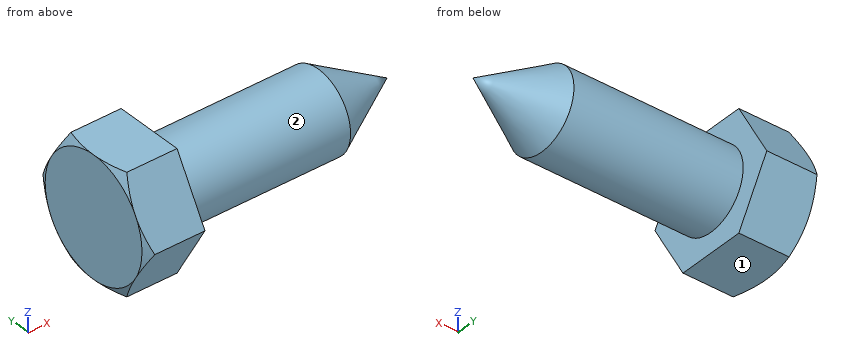
```python
from build123d import *

# Parameters (mm, degrees)
BASEHEAD_DEPTH = 17.78


with BuildPart() as part:
    # Sketch1 → BaseHead (new body)
    with BuildSketch(Plane(origin=(0, 0, 0), x_dir=(0, 0, -1), z_dir=(1, 0, 0))):
        Polygon((19.05, 10.998522628), (19.05, -10.998522628), (0, -21.997045256), (-19.05, -10.998522628), (-19.05, 10.998522628), (0, 21.997045256), align=None)
    extrude(amount=BASEHEAD_DEPTH)

    # Sketch2 → BaseBody (revolve)
    with BuildSketch(Plane.XY, mode=Mode.PRIVATE) as basebody_sk:
        Polygon((0, 0), (93.98, 0), (71.982954744, 12.7), (0, 12.7), align=None)
    revolve(basebody_sk.sketch.rotate(Axis((0, 0, 0), (1, 0, 0)), 90), axis=Axis((0, 0, 0), (1, 0, 0)))

    # Sketch3 → HeadChamfer (revolve, cut)
    with BuildSketch(Plane.XY):
        Polygon((0, 19.05), (5.367651581, 28.347045256), (5.367651581, 34.697045256), (-12.7, 34.697045256), (-12.7, 19.05), align=None)
    revolve(axis=Axis((0, 0, 0), (1, 0, 0)), mode=Mode.SUBTRACT)


solid = part.part
```
Input: part model. Units: mm. Frame: model coordinates. Face numbers are marked on the shaded views. A direction names the side the tool comes from. Coordinates: 2 decimals unless noted, no trailing zeros. Write each loop counter-clockwise with the first axis right and the second up, starting at its lowest first coordinate (ties: lowest second). Pieces come first, ordered by that corner, then holes. Notation, with made-up numbers: M -22,-13 L 22,-13 A10 ccw 22,-8 Z; hole C 78.25,-15 d2. An arc over 180 degrees is marked long. Use one line per item in the form item = value.
Q1. First-contact query: pin 1 (1.5 mm diameter, centred on x = 36.5, y = 2.5, fed in from +Z); pin 2 (5 mm diameter, centred on x = 75, z = -7, fed in from +Y); pin 3 (19 mm diameter, centred on y = 6.5, z = -8.5, fed in from +X). Flat tips, straight axial feed; report the tip coordinate or a pass-through.
Answer below:
pin_1 = 12.58
pin_2 = 10.79
pin_3 = 91.9
Q2. Section B-B (x = 87.5). Return loops of the section in (y, z).
Answer below:
outline = C 0,0 d7.48
Q3. Section A-A (x = 66.5). Return loops of the section in (y, z), plus the area to 3 significant figures.
Answer below:
outline = C 0,0 d25.4
area = 507 mm²
Q4. Material intervals for probe 1 along X at (y, z) = (11, -7); probe 2 along Y at (x, z) = (66.5, 9); probe 3 along Z at (x, y) = (30.5, 2.5), sorted ascending. Write a range as from..to.
Answer below:
probe_1 = 0..17.78
probe_2 = -8.96..8.96
probe_3 = -12.45..12.45
Q5. Set-up query: the marked faces 1 and 2. Return all of +Z, -Z, +X, -X, +Y, -Y with unobstructed straight access to the full face (end or side cutting, diameter ignored); none if empty.
Answer below:
face_1 = -Z, +X, -X, +Y, -Y
face_2 = +X
